```python
from build123d import *

# Parameters (mm, degrees)
F0_R     = 2.778125
F1_DEPTH = 1.3890625
F2_R     = 1.3890625
F3_DEPTH = 12.7
F4_W     = 0.79375
F4_H     = 3.175
F6_DEPTH = 2.38125
F5_W     = 3.175
F5_H     = 0.79375
F7_DEPTH = 2.38125
F8_R     = 0.127
F10_SIZE = 1.3335


# Not quite as in the source:
# - a fillet or chamfer that OpenCascade refuses, or shapes differently, is made with other operations: its cross-section is extruded or revolved along the edge and cut away or added


with BuildPart() as f1:
    # F0 (on Front) → F1 (new body, symmetric)
    with BuildSketch(Plane.XZ):
        Circle(F0_R)
    extrude(amount=F1_DEPTH, both=True)

    # F2 (on face) → F3 (join)
    with BuildSketch(Plane.XZ.offset(1.3890625)):
        Circle(F2_R)
    extrude(amount=F3_DEPTH)

    # F4 (on face) → F6 (cut)
    with BuildSketch(Plane(origin=(0, 1.3890625, 0), x_dir=(-1, 0, 0), z_dir=(0, 1, 0))):
        Rectangle(F4_W, F4_H)
    extrude(amount=-F6_DEPTH, mode=Mode.SUBTRACT)

    # F5 (on face) → F7 (cut)
    with BuildSketch(Plane(origin=(0, 1.3890625, 0), x_dir=(-1, 0, 0), z_dir=(0, 1, 0))):
        Rectangle(F5_W, F5_H)
    extrude(amount=-F7_DEPTH, mode=Mode.SUBTRACT)

    # F8
    f8_edges = [f1.edges().sort_by_distance(p)[0] for p in [
        (0.396875, 0.198438, 0.396875),
        (-0.396875, 0.198438, 0.396875),
        (-0.396875, 0.198438, -0.396875),
        (0.396875, 0.198438, -0.396875),
    ]]
    fillet(f8_edges, radius=F8_R)

    # F9: fillet of radius 1.27 on 1 edges, made by hand

    # F9_s1 → F9_t2 (revolve, cut)
    with BuildSketch(Plane.XY):
        with BuildLine():
            ThreePointArc((1.508125, 1.3890625), (2.4061506121, 1.0170881121), (2.778125, 0.1190625))
            Line((2.778125, 0.1190625), (2.778125, 1.3890625))
            Line((2.778125, 1.3890625), (1.508125, 1.3890625))
        make_face()
    revolve(axis=Axis((0, 1.3890625, 0), (0, -1, 0)), mode=Mode.SUBTRACT)

    # F10
    f10_edges = [f1.edges().sort_by_distance(p)[0] for p in [
        (-1.389062, -14.089062, 0),
    ]]
    chamfer(f10_edges, length=F10_SIZE)


solid = f1.part
```
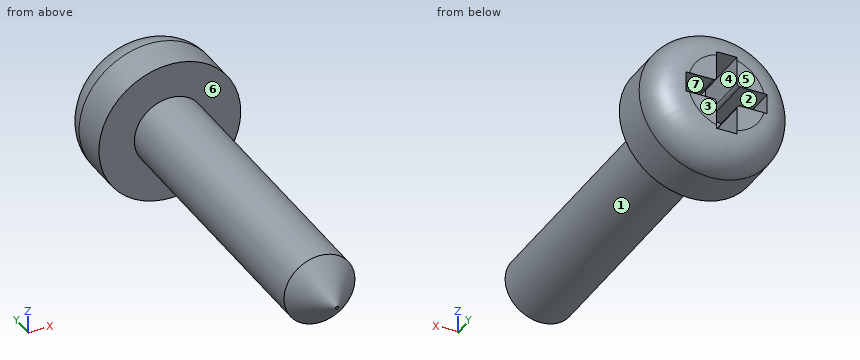
CAD build for the part. Positions are in the model's coordinates, mm. Face numbers are marked on the shaded views. A direction names the side the tool comes from. Round coordinates to 2 decimals unless told otherwise and drop trailing zeros. Write each loop counter-clockwise with the first axis right and the second up, starting at its lowest first coordinate (ties: lowest second). Pieces come first, ordered by that corner, then holes. Notation, with made-up numbers: (-7.75, 86.25) -> (43.25, 86.25) arc R14 cw to (43.25, 91.25) -> close; hole circle Ø4 at (-32, 45). An arc over 180 degrees is marked (long way). Answer in a Markdown table with one row per item. Add a question column.
Item 1: Saw through at A-A, the plane y = -3.5. Write the cut outline in (x, z).
Item 2: Which spindle directions (+Z, -Z, +X, -X, +Y, -Y) get a long thin tool onto all of the face, cutting with end or side? Do the marked faces 5, 6 and 7. Say none if no direction does.
Item 3: Drop flat-ended pins along their axis: pin 1 Ø0.5 at (y, z) = (-0.5, -1) entering from -X (3 decimals); pin 2 Ø0.5 at (y, z) = (0, 1) entering from +X (3 decimals); pin 3 Ø0.5 at (x, y) = (-1, -0.5) entering from +Z (3 decimals). Give the stop position or say it passes through.
Item 4: Drill centre lines: line 1 (X direction, y = 0, z = -0.15); line 2 (Y direction, x = -1.2, z = 0.75). Where is each one in solid material? Low to high. Write a range as from..to.
Item 5: Mould opens along X. For the marked faces 1, 2, 3 and 4 say: pulls with the +X half, pulls with the -X half, needs draft (parallel to the pull), parting line crosses it, or undercut.
Findings below:
| question | item | result |
|---|---|---|
| 1 | outline | circle Ø2.78 at (0, 0) |
| 2 | face 5 | +Z, -Z, +X, -X, +Y |
| 2 | face 6 | -Y |
| 2 | face 7 | +Y |
| 3 | pin 1 | stops at x = -2.675 |
| 3 | pin 2 | stops at x = 2.675 |
| 3 | pin 3 | stops at z = 2.675 |
| 4 | line 1 | x = -2.77..-1.59, 1.59..2.77 |
| 4 | line 2 | y = -1.39..1.39 |
| 5 | face 1 | parting line crosses it |
| 5 | face 2 | undercut |
| 5 | face 3 | needs draft |
| 5 | face 4 | undercut |
